```python
from build123d import *

# Parameters (mm, degrees)
F0_R         = 0.4976358306
F4_DEPTH     = 17.4
F5_T1_DEPTH  = 145.6880456822
F5_T3_DEPTH  = 145.6880456822
F5_T5_DEPTH  = 145.6880456822
F5_T7_DEPTH  = 145.6880456822
F5_T9_DEPTH  = 145.6880456822
F5_T11_DEPTH = 145.6880456822
F7_DEPTH     = 0.8


# Not quite as in the source:
# - a fillet or chamfer that OpenCascade refuses, or shapes differently, is made with other operations: its cross-section is extruded or revolved along the edge and cut away or added


with BuildPart() as f3:
    # F2 (on offset) → F3 section 0
    with BuildSketch(Plane.XY.offset(48)):
        Polygon((21.4103630818, 51.6891889274), (-21.4103630818, 51.6891889274), (-51.6891889274, 21.4103630818), (-51.6891889274, -21.4103630818), (-21.4103630818, -51.6891889274), (21.4103630818, -51.6891889274), (51.6891889274, -21.4103630818), (51.6891889274, 21.4103630818), align=None)
    # F0 (on Top) → F3 section 1
    with BuildSketch(Plane.XY):
        Circle(F0_R)
    loft()

    # F4 (add): a face of the model
    f4_faces = [f3.faces().sort_by_distance(p)[0] for p in [
        (0, 0, 48),
    ]]
    extrude(f4_faces, amount=F4_DEPTH)

    # F5: chamfer of 20 on 8 edges, made by hand

    # F5_s2 → F5_t1 (cut)
    with BuildSketch(Plane(origin=(-51.5085025199, -51.5085025199, 0), x_dir=(0, 0, 1), z_dir=(0.7071067812, 0.7071067812, 0))):
        Polygon((45.4, 51.6891889274), (65.4, 31.6891889274), (65.4, 51.6891889274), align=None)
    extrude(amount=F5_T1_DEPTH, mode=Mode.SUBTRACT)

    # F5_s4 → F5_t3 (cut)
    with BuildSketch(Plane.YZ.offset(-72.8440228411)):
        Polygon((-31.6891889274, 65.4), (-51.6891889274, 45.4), (-51.6891889274, 65.4), align=None)
        Polygon((31.6891889274, 65.4), (51.6891889274, 45.4), (51.6891889274, 65.4), align=None)
    extrude(amount=F5_T3_DEPTH, mode=Mode.SUBTRACT)

    # F5_s6 → F5_t5 (cut)
    with BuildSketch(Plane(origin=(-51.5085025199, 51.5085025199, 0), x_dir=(0, 0, 1), z_dir=(0.7071067812, -0.7071067812, 0))):
        Polygon((65.4, 31.6891889274), (45.4, 51.6891889274), (65.4, 51.6891889274), align=None)
    extrude(amount=F5_T5_DEPTH, mode=Mode.SUBTRACT)

    # F5_s8 → F5_t7 (cut)
    with BuildSketch(Plane.XZ.offset(-72.8440228411)):
        Polygon((51.6891889274, 45.4), (31.6891889274, 65.4), (51.6891889274, 65.4), align=None)
        Polygon((-31.6891889274, 65.4), (-51.6891889274, 45.4), (-51.6891889274, 65.4), align=None)
    extrude(amount=F5_T7_DEPTH, mode=Mode.SUBTRACT)

    # F5_s10 → F5_t9 (cut)
    with BuildSketch(Plane(origin=(51.5085025199, 51.5085025199, 0), x_dir=(0, 0, 1), z_dir=(-0.7071067812, -0.7071067812, 0))):
        Polygon((65.4, 31.6891889274), (45.4, 51.6891889274), (65.4, 51.6891889274), align=None)
    extrude(amount=F5_T9_DEPTH, mode=Mode.SUBTRACT)

    # F5_s12 → F5_t11 (cut)
    with BuildSketch(Plane(origin=(51.5085025199, -51.5085025199, 0), x_dir=(0, 0, 1), z_dir=(-0.7071067812, 0.7071067812, 0))):
        Polygon((65.4, 31.6891889274), (45.4, 51.6891889274), (65.4, 51.6891889274), align=None)
    extrude(amount=F5_T11_DEPTH, mode=Mode.SUBTRACT)

    # F6 (on face) → F7 (cut)
    with BuildSketch(Plane(origin=(-34.3262119352, 34.3262119352, 48.5445944637), x_dir=(0.8660254038, 0.2886751346, 0.4082482905), z_dir=(-0.5, 0.5, 0.7071067812))):
        Polygon((20.256810503, -7.3152106315), (21.0549216717, -6.755489856), (16.5048241615, 1.810487709), (11.6832025843, -0.902343074), (12.6268315784, -1.8886970465), (15.5827937516, 0), align=None)
        Polygon((7.1851625107, -3.7115143208), (8.0320088518, -4.8281169212), (11.6832025843, -11.3175281272), (13.5610239533, -10.2609931974), (9.3989199392, -4.8281169212), (10.6345172528, -3.6460408281), (14.9572589197, -9.2744808388), (16.3466744125, -8.9773000983), (10.7584019824, -1.7010715934), align=None)
        Polygon((6.170399487, -11.8845931934), (9.7690848634, -11.8845931934), (4.6387440525, -3.8551988546), (1.9462815717, -6.7955303045), align=None)
        Polygon((4.0612965822, -7.0431958884), (4.5432327315, -6.7955303045), (7.355309773, -10.5520610512), (6.8237950711, -10.8511117796), align=None, mode=Mode.SUBTRACT)
        Polygon((7.1851625107, -16.2641853094), (6.7229871638, -14.1033669934), (0.7042393052, -8.0728225242), (4.2175897397, -16.8479587883), (5.6911348405, -15.9064446157), (3.3750016382, -12.2815106186), align=None)
        Polygon((2.9365293457, -17.6483038813), (4.5432327315, -17.9625210545), (-2.3575761854, -8.9773000983), (-3.3578095237, -9.7454970267), align=None)
        Polygon((0.946887175, -20.9094267339), (-1.3764705509, -20.9094267339), (-1.3764705509, -22.1590939909), (1.3320371509, -21.1326684803), (2.4291982409, -17.6483038813), (-3.3762898288, -10.2609931974), (-7.2390597263, -13.7484027895), (-8.7199002404, -12.10817499), (-9.5777362585, -12.8826517612), (-8.4756426513, -14.1033669934), (-5.128640122, -17.7334435545), (-3.6981627345, -16.819447279), (-2.2488206246, -15.5000568389), (-3.1974268837, -14.4016498716), (-4.9229765081, -15.8918690917), (-6.4675627457, -14.1033669934), (-3.5124101047, -11.5512379779), (1.7531381398, -17.6483038813), align=None)
    extrude(amount=-F7_DEPTH, mode=Mode.SUBTRACT)


solid = f3.part
```
For this review, take the finished solid that the model builds, in its own axes (mm). A direction names the side the tool comes from. Round coordinates to 2 decimals unless told otherwise and drop trailing zeros. Use one line per item in the form item = value.
Q1. To check wall thickness, follow probe 1 along X at (y, z) = (38, 43); probe 2 along X at (y, z) = (9.5, 23); probe 3 along Z at (x, y) = (25, 4.5). State the ranges of each line that lie inside material, in increasing order. Write a range as from..to.
Resolved:
probe_1 = -27.56..27.56
probe_2 = -25.01..25.01
probe_3 = 22.98..65.4
Q2. Clearance check with flat-ended pins moving along their axes: pin 1 Ø10 at (y, z) = (27.5, 37.5) entering from -X; pin 2 Ø8 at (y, z) = (7.5, 34) entering from +X; pin 3 Ø1 at (y, z) = (-0.5, 32) entering from -X. State where each tip first meets the part, or that it passes through.
Resolved:
pin_1 = -38.81
pin_2 = 41.02
pin_3 = -35.16
Q3. Machinability: for faces 1 (the flat face through (-21.932, 37.413, 54.568)), 2 (the flat face through (-29.36, 28.78, 55.98)), 3 (the flat face through (-19.17, 37.44, 55.93)), which of the approach directions +Z, -Z, +X, -X, +Y, -Y give a long, thin tool a straight path to every point of the face, cutting with its end or side? Answer none if there is none.
Resolved:
face_1 = +Y
face_2 = +Z, -X, +Y
face_3 = none
Q4. The part is to be moulded in two halves that separate along Z. For faces 4 (the flat face through (-34.35, 22.92, 56.04)), 5 (the flat face through (-37.046, 20.033, 55.597)), 6 (the flat face through (-0.29, -40.89, 56.2)), say which applies: released by +Z, released by -Z, zero draft, split by the parting line, or undercut.
Resolved:
face_4 = undercut
face_5 = undercut
face_6 = released by +Z
